Work out the finished part from the listing and answer in its coordinate system (mm). A direction names the side the tool comes from. Round coordinates to 2 decimals unless told otherwise and drop trailing zeros. Order: outer loops, then holes, each group sorted by start corner. A loop starts at its lowest first (then second) coordinate and runs counter-clockwise, first axis right, second up. Notation, with made-up numbers: M 44,-6 L 87,-6 A24 ccw 87,29 Z; hole C 66.25,49.25 d8. An arc over 180 degrees is marked long. Return JSON: item names as keys, results as strings.
from build123d import *

# Parameters (mm, degrees)
BOSS_EXTRUDE1_DEPTH     = 100
BOSS_EXTRUDE2_DEPTH     = 15
SKETCH3_W               = 25
SKETCH3_H               = 40
CUT_EXTRUDE1_DEPTH      = 21
CUT_EXTRUDE1_DEPTH_BACK = 60.25
SKETCH4_W               = 20
SKETCH4_H               = 15
BOSS_EXTRUDE3_DEPTH     = 55
SKETCH5_W               = 20
SKETCH5_H               = 15
BOSS_EXTRUDE4_DEPTH     = 40
CUT_EXTRUDE2_DEPTH      = 60.5
CUT_EXTRUDE2_DEPTH_BACK = 55.672438422


with BuildPart() as part:
    # Sketch1 → Boss-Extrude1 (new body)
    with BuildSketch(Plane.XY):
        with BuildLine():
            Line((-10, 58.400021404), (-10, 43.400021404))
            Line((-10, 43.400021404), (-25, 43.400021404))
            Line((-25, 43.400021404), (-25, 28.400021404))
            Line((-25, 28.400021404), (-10, 28.400021404))
            Line((-10, 28.400021404), (-10, 8.900021404))
            ThreePointArc((-10, 8.900021404), (-7.071067812, 1.828953592), (0, -1.099978596))
            Line((0, -1.099978596), (20, -1.099978596))
            Line((20, -1.099978596), (20, -16.099978596))
            Line((20, -16.099978596), (-20, -16.099978596))
            Line((-20, -16.099978596), (-20, -55.772417018))
            ThreePointArc((-20, -55.772417018), (-59.024032595, 5.169726898), (-10, 58.400021404))
        make_face()
    extrude(amount=-BOSS_EXTRUDE1_DEPTH)

    # Sketch2 → Boss-Extrude2 (add)
    with BuildSketch(Plane.XY):
        with BuildLine():
            Line((20, -11.099978596), (-58.976442171, 5.686982405))
            ThreePointArc((-58.976442171, 5.686982405), (-50.036327292, -31.732135938), (-20, -55.772417018))
            Line((-20, -55.772417018), (-20, -16.099978596))
            Line((-20, -16.099978596), (20, -16.099978596))
            Line((20, -16.099978596), (20, -11.099978596))
        make_face()
    extrude(amount=BOSS_EXTRUDE2_DEPTH)

    # Sketch3 → Cut-Extrude1 (cut, two sides)
    with BuildSketch(Plane(origin=(0, 0, 0), x_dir=(0, 0, -1), z_dir=(1, 0, 0))) as cut_extrude1_sk:
        with Locations((42.5, 38.400021404)):
            Rectangle(SKETCH3_W, SKETCH3_H)
    extrude(amount=CUT_EXTRUDE1_DEPTH, mode=Mode.SUBTRACT)
    extrude(cut_extrude1_sk.sketch, amount=-CUT_EXTRUDE1_DEPTH_BACK, mode=Mode.SUBTRACT)

    # Sketch4 → Boss-Extrude3 (add)
    with BuildSketch(Plane.XY.offset(-55)):
        with Locations((-15, 35.900021404)):
            Rectangle(SKETCH4_W, SKETCH4_H)
    extrude(amount=-BOSS_EXTRUDE3_DEPTH)

    # Sketch5 → Boss-Extrude4 (add)
    with BuildSketch(Plane(origin=(0, 0, -30), x_dir=(-1, 0, 0), z_dir=(0, 0, -1))):
        with Locations((15, 35.900021404)):
            Rectangle(SKETCH5_W, SKETCH5_H)
    extrude(amount=-BOSS_EXTRUDE4_DEPTH)

    # Sketch6 → Cut-Extrude2 (cut, two sides)
    with BuildSketch(Plane(origin=(0, -1.099978596, 0), x_dir=(1, 0, 0), z_dir=(0, 1, 0))) as cut_extrude2_sk:
        with BuildLine():
            Line((15, 90), (15, 10))
            ThreePointArc((15, 10), (10, 5), (5, 10))
            Line((5, 10), (5, 90))
            ThreePointArc((5, 90), (10, 95), (15, 90))
        make_face()
    extrude(amount=CUT_EXTRUDE2_DEPTH, mode=Mode.SUBTRACT)
    extrude(cut_extrude2_sk.sketch, amount=-CUT_EXTRUDE2_DEPTH_BACK, mode=Mode.SUBTRACT)


solid = part.part
Item 1: Find section C-C (y = 45). Determine the outline of the cut face in (x, z), plus the area to 3 significant figures.
Output:
{"outline": "M -38.54,-100 L -10,-100 L -10,-55 L -38.54,-55 Z; M -38.54,-30 L -10,-30 L -10,0 L -38.54,0 Z", "area": "2,140 mm^2"}
Item 2: Find section D-D (x = -41). Determine the outline of the cut face in (y, z).
Output:
{"outline": "M -42.77,-100 L 42.77,-100 L 42.77,-55 L 18.4,-55 L 18.4,-30 L 42.77,-30 L 42.77,0 L 1.87,0 L 1.87,15 L -42.77,15 Z"}
Item 3: Consider line 1 along X through (y, z) = (-9.5, -53.5); line 2 along X through (y, z) = (-3.5, -79); line 3 along Y through (x, z) = (-9, -84). Determine where each line is inside the solid, lowest interval first. Write a range as [from, to].
Output:
{"line 1": "x = [-58.48, 5], [15, 20]", "line 2": "x = [-59.15, 5], [15, 20]", "line 3": "y = [-16.1, 4.54], [28.4, 43.4]"}
Item 4: Find section A-A (z = -59). Determine the outline of the cut face in (x, y), plus the area to 3 significant figures.
Output:
{"outline": "M -20,-55.77 L -20,-16.1 L 5,-16.1 L 5,-1.1 L 0,-1.1 A10 cw -10,8.9 L -10,28.4 L -5,28.4 L -5,43.4 L -10,43.4 L -10,58.4 A59.25 ccw Z; M 15,-16.1 L 20,-16.1 L 20,-1.1 L 15,-1.1 Z", "area": "4,320 mm^2"}
Item 5: Each of these flat-tipped pins is pushed along its axis until it touches: pin 1 (12 mm diameter, centred on y = -29, z = -69, fed in from +X); pin 2 (1.5 mm diameter, centred on y = 46, z = -56, fed in from -X); pin 3 (10 mm diameter, centred on x = -17.5, z = -18, fed in from +Y). Where does it stop, or does it pass through?
Output:
{"pin 1": "stops at x = -20", "pin 2": "stops at x = -38.25", "pin 3": "stops at y = 57.92"}
Item 6: Find section B-B (x = 7). Determine the outline of the cut face in (y, z), plus the area to 3 significant figures.
Output:
{"outline": "M -16.1,-100 L -1.1,-100 L -1.1,-94 L -16.1,-94 Z; M -16.1,-6 L -1.1,-6 L -1.1,0 L -8.34,0 L -8.34,15 L -16.1,15 Z", "area": "296 mm^2"}
Item 7: The mould has two halves that part along X. Classify faces 1 (the flat face through (-25, 36, 5)), 2 (the flat face through (0, -16.1, -43)), 3 (the cylindrical face through (10, -8, -5)): pulls with the +X half, pulls with the -X half, needs draft (parallel to the pull), parting line crosses it, or undercut.
Output:
{"face 1": "pulls with the -X half", "face 2": "needs draft", "face 3": "undercut"}
Item 8: Which of the six approach directions +Z, -Z, +X, -X, +Y, -Y give full straight-line access (tool end or side, diameter ignored) to faces 4 (the flat face through (-5, 36, -82)), 5 (the flat face through (-25, 36, -105)), 6 (the flat face through (-8, 43.4, -94)), 7 (the cylindrical face through (10, -8, -95)), 8 (the flat face through (-33, 18.4, -42))?
Output:
{"face 4": "+Z, -Z, +X, +Y", "face 5": "-Z, -X, +Y, -Y", "face 6": "-Z, +X, +Y", "face 7": "+Y, -Y", "face 8": "+X, -X, +Y"}
